CAD build for the part. Positions are in the model's coordinates, mm. Face numbers are marked on the shaded views. Give positions to 0.01 mm unless a question says otherwise; leave off trailing zeros. Loops run counter-clockwise (first coordinate to the right, second up) from the corner with the lowest first, then second, coordinate; pieces in that order, holes last. Notation, with made-up numbers: (-19.5, -38) - (32.5, -38) arc R19 cw to (32.5, -26) - close; hole circle Ø2 at (-15, 28.25). An arc over 180 degrees is marked (long way). Return JSON: item names as keys, results as strings.
from build123d import *

# Parameters (mm, degrees)
F0_W          = 7
F0_H          = 6.5
F0_W_2        = 13.5
F0_H_2        = 21
F0_R          = 1.2
F1_DEPTH      = 10
F1_FACE_W     = 27.5
F1_FACE_H     = 34
F2_DEPTH      = 0.5
F3_DEPTH      = 1
F4_DEPTH      = 8
F4_DEPTH_BACK = 1
F6_DEPTH      = 34.001


with BuildPart() as f1:
    # F0 (on Front) → F1 (new body)
    with BuildSketch(Plane.XZ):
        with Locations((-49.9074855894, 34.1609876885)):
            Rectangle(F0_W, F0_H)
        with Locations((-39.6574855894, 34.1609876885)):
            Rectangle(F0_W_2, F0_H)
        with Locations((-49.9074855894, 20.4109876885)):
            Rectangle(F0_W, F0_H_2)
        with Locations((-49.6574855894, 12.9109876885)):
            Circle(F0_R, mode=Mode.SUBTRACT)
        with Locations((-49.6574855894, 27.9109876885)):
            Circle(F0_R, mode=Mode.SUBTRACT)
        with Locations((-29.4074855894, 34.1609876885)):
            Rectangle(F0_W, F0_H)
        with Locations((-49.9074855894, 6.6609876885)):
            Rectangle(F0_W, F0_H)
        with Locations((-29.4074855894, 20.4109876885)):
            Rectangle(F0_W, F0_H_2)
        with Locations((-29.6574855894, 12.9109876885)):
            Circle(F0_R, mode=Mode.SUBTRACT)
        with Locations((-29.6574855894, 27.9109876885)):
            Circle(F0_R, mode=Mode.SUBTRACT)
        with Locations((-39.6574855894, 6.6609876885)):
            Rectangle(F0_W_2, F0_H)
        with Locations((-29.4074855894, 6.6609876885)):
            Rectangle(F0_W, F0_H)
        with Locations((-39.6574855894, 20.4109876885)):
            Rectangle(F0_W_2, F0_H_2)
        with Locations((-49.6574855894, 27.9109876885)):
            Circle(F0_R)
        with Locations((-49.6574855894, 12.9109876885)):
            Circle(F0_R)
        with Locations((-29.6574855894, 12.9109876885)):
            Circle(F0_R)
        with Locations((-29.6574855894, 27.9109876885)):
            Circle(F0_R)
    extrude(amount=F1_DEPTH)

    # F0 (on Front) + F1_face (on face) → F2 (join)
    with BuildSketch(Plane.XZ):
        with Locations((-49.9074855894, 34.1609876885)):
            Rectangle(F0_W, F0_H)
        with Locations((-39.6574855894, 34.1609876885)):
            Rectangle(F0_W_2, F0_H)
        with Locations((-49.9074855894, 20.4109876885)):
            Rectangle(F0_W, F0_H_2)
        with Locations((-49.6574855894, 12.9109876885)):
            Circle(F0_R, mode=Mode.SUBTRACT)
        with Locations((-49.6574855894, 27.9109876885)):
            Circle(F0_R, mode=Mode.SUBTRACT)
        with Locations((-29.4074855894, 34.1609876885)):
            Rectangle(F0_W, F0_H)
        with Locations((-49.9074855894, 6.6609876885)):
            Rectangle(F0_W, F0_H)
        with Locations((-29.4074855894, 20.4109876885)):
            Rectangle(F0_W, F0_H_2)
        with Locations((-29.6574855894, 12.9109876885)):
            Circle(F0_R, mode=Mode.SUBTRACT)
        with Locations((-29.6574855894, 27.9109876885)):
            Circle(F0_R, mode=Mode.SUBTRACT)
        with Locations((-39.6574855894, 6.6609876885)):
            Rectangle(F0_W_2, F0_H)
        with Locations((-29.4074855894, 6.6609876885)):
            Rectangle(F0_W, F0_H)
        with Locations((-29.6574855894, 27.9109876885)):
            Circle(F0_R)
        with Locations((-49.6574855894, 27.9109876885)):
            Circle(F0_R)
        with Locations((-49.6574855894, 12.9109876885)):
            Circle(F0_R)
        with Locations((-29.6574855894, 12.9109876885)):
            Circle(F0_R)
    with BuildSketch(Plane(origin=(-39.6574855894, -10, 20.4109876885), x_dir=(1, 0, 0), z_dir=(0, -1, 0))):
        Rectangle(F1_FACE_W, F1_FACE_H)
    extrude(amount=-F2_DEPTH)

    # F0 (on Front) → F3 (cut)
    with BuildSketch(Plane.XZ):
        with Locations((-29.4074855894, 34.1609876885)):
            Rectangle(F0_W, F0_H)
        with Locations((-39.6574855894, 34.1609876885)):
            Rectangle(F0_W_2, F0_H)
        with Locations((-49.9074855894, 34.1609876885)):
            Rectangle(F0_W, F0_H)
        with Locations((-49.9074855894, 6.6609876885)):
            Rectangle(F0_W, F0_H)
        with Locations((-39.6574855894, 6.6609876885)):
            Rectangle(F0_W_2, F0_H)
        with Locations((-29.4074855894, 6.6609876885)):
            Rectangle(F0_W, F0_H)
    extrude(amount=-F3_DEPTH, mode=Mode.SUBTRACT)

    # F0 (on Front) → F4 (cut, two sides)
    with BuildSketch(Plane.XZ) as f4_sk:
        with Locations((-29.6574855894, 27.9109876885)):
            Circle(F0_R)
        with Locations((-29.6574855894, 12.9109876885)):
            Circle(F0_R)
        with Locations((-49.6574855894, 12.9109876885)):
            Circle(F0_R)
        with Locations((-49.6574855894, 27.9109876885)):
            Circle(F0_R)
    extrude(amount=F4_DEPTH, mode=Mode.SUBTRACT)
    extrude(f4_sk.sketch, amount=-F4_DEPTH_BACK, mode=Mode.SUBTRACT)

    # F5 (on face) → F6 (cut, through all)
    with BuildSketch(Plane(origin=(0, 0, 3.4109876885), x_dir=(1, 0, 0), z_dir=(0, 0, -1))):
        with BuildLine():
            Line((-33.6574855894, 8.5455439207), (-33.6574855894, 10))
            Line((-33.6574855894, 10), (-45.6574855894, 10))
            Line((-45.6574855894, 10), (-45.6574855894, 8.5455439207))
            ThreePointArc((-45.6574855894, 8.5455439207), (-44.6894279438, 7.7187269742), (-45.0574855894, 6.5))
            Line((-45.0574855894, 6.5), (-45.0574855894, 5.5))
            Line((-45.0574855894, 5.5), (-34.2574855894, 5.5))
            Line((-34.2574855894, 5.5), (-34.2574855894, 6.5))
            ThreePointArc((-34.2574855894, 6.5), (-34.6099684918, 7.7141585825), (-33.6574855894, 8.5455439207))
        make_face()
    extrude(amount=-F6_DEPTH, mode=Mode.SUBTRACT)


solid = f1.part
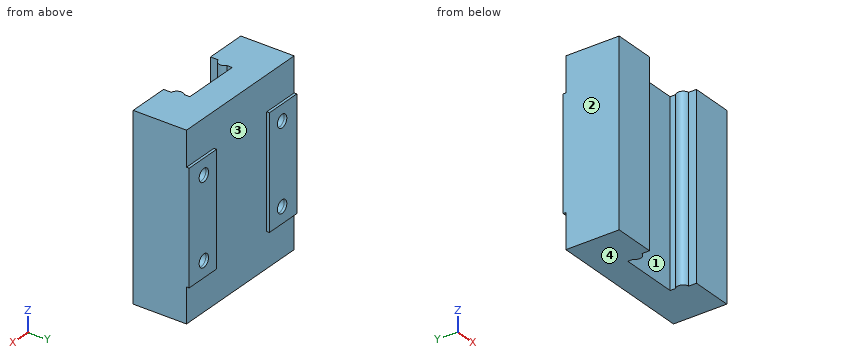
1. Cut at D-D, the plane z = 18.5. Write the cut outline in (x, y), plus the area to 3 significant figures.
Values follow:
{"outline": "(-53.41, -10) - (-45.66, -10) - (-45.66, -8.55) arc R1.16 ccw to (-45.06, -6.5) - (-45.06, -5.5) - (-34.26, -5.5) - (-34.26, -6.5) arc R1.18 ccw to (-33.66, -8.55) - (-33.66, -10) - (-25.91, -10) - (-25.91, 0.5) - (-32.91, 0.5) - (-32.91, 0) - (-46.41, 0) - (-46.41, 0.5) - (-53.41, 0.5) - close", "area": "233 mm²"}
2. Cut at A-A, the plane z = 5. Write the cut outline in (x, y).
Values follow:
{"outline": "(-53.41, -10) - (-45.66, -10) - (-45.66, -8.55) arc R1.16 ccw to (-45.06, -6.5) - (-45.06, -5.5) - (-34.26, -5.5) - (-34.26, -6.5) arc R1.18 ccw to (-33.66, -8.55) - (-33.66, -10) - (-25.91, -10) - (-25.91, 0) - (-53.41, 0) - close"}
3. Drop flat-ended pins along their axis: P1, Ø12, axis at x = -35.5, z = 30, coming from the +Y side; P2, Ø1.2, axis at x = -50, z = 12.5, coming from the +Y side; P3, Ø1, axis at x = -36.5, z = 10.5, coming from the -Y side. Give the stop position or say it passes through.
Values follow:
{"P1": "stops at y = 0.5", "P2": "stops at y = -8", "P3": "stops at y = -5.5"}
4. Cut at C-C, the plane y = -3.5. Write the cut outline in (x, z), plus the area to 3 significant figures.
Values follow:
{"outline": "(-53.41, 3.41) - (-25.91, 3.41) - (-25.91, 37.41) - (-53.41, 37.41) - close; hole circle Ø2.4 at (-49.66, 12.91); hole circle Ø2.4 at (-49.66, 27.91); hole circle Ø2.4 at (-29.66, 12.91); hole circle Ø2.4 at (-29.66, 27.91)", "area": "917 mm²"}
5. Drill centre lines: probe 1 along X at (y, z) = (-3.25, 28.5); probe 2 along X at (y, z) = (-7.5, 8.5); probe 3 along X at (y, z) = (-9, 8.5). Where is each one in solid material? Low to high.
Values follow:
{"probe 1": "x = -53.41 to -50.7, -48.61 to -30.7, -28.61 to -25.91", "probe 2": "x = -53.41 to -44.65, -34.65 to -25.91", "probe 3": "x = -53.41 to -45.66, -33.66 to -25.91"}
6. Pull direction X, two halves, no side cores. Call the marked faces 1, 2, 3 and 4: +X half, -X half, draft (parallel to the pull), parting line (faces both ways), or undercut.
Values follow:
{"face 1": "undercut", "face 2": "-X half", "face 3": "undercut", "face 4": "draft"}
7. Cut at B-B, the plane x = -48. Write the cut outline in (y, z), plus the area to 4 significant figures.
Values follow:
{"outline": "(-10, 3.41) - (0, 3.41) - (0, 9.91) - (0.5, 9.91) - (0.5, 30.91) - (0, 30.91) - (0, 37.41) - (-10, 37.41) - close", "area": "350.5 mm²"}
